from build123d import *

# Parameters (mm, degrees)
F1_DEPTH = 90.3440154
F2_R     = 2.0828
F3_DEPTH = 3.175
F5_DEPTH = 20.240498
F6_SIZE  = 20.240488
F7_R     = 1.7272
F8_DEPTH = 4.7625


# Not quite as in the source:
# - a fillet or chamfer is up to 0.001 mm smaller than in the source, because OpenCascade refuses the exact size


with BuildPart() as f1:
    # F0 (on Top) → F1 (new body)
    with BuildSketch(Plane.XY):
        with BuildLine():
            Line((32.7249998, 0), (0, 0))
            Line((0, 0), (0, 1.1500104))
            ThreePointArc((0, 1.1500104), (-10.675, 11.8250104), (-21.35, 1.1500104))
            Line((-21.35, 1.1500104), (-21.35, -3.175))
            Line((-21.35, -3.175), (-18.175, -3.175))
            Line((-18.175, -3.175), (-18.175, 1.1500104))
            ThreePointArc((-18.175, 1.1500104), (-10.675, 8.6500104), (-3.175, 1.1500104))
            Line((-3.175, 1.1500104), (-3.175, -3.175))
            Line((-3.175, -3.175), (35.8999998, -3.175))
            Line((35.8999998, -3.175), (35.8999998, 1.1500104))
            ThreePointArc((35.8999998, 1.1500104), (43.3999998, 8.6500104), (50.8999998, 1.1500104))
            Line((50.8999998, 1.1500104), (50.8999998, -3.175))
            Line((50.8999998, -3.175), (54.0749998, -3.175))
            Line((54.0749998, -3.175), (54.0749998, 1.1500104))
            ThreePointArc((54.0749998, 1.1500104), (43.3999998, 11.8250104), (32.7249998, 1.1500104))
            Line((32.7249998, 1.1500104), (32.7249998, 0))
        make_face()
    extrude(amount=F1_DEPTH)

    # F2 (on face) → F3 (cut, through all)
    with BuildSketch(Plane(origin=(0, 0, 0), x_dir=(-1, 0, 0), z_dir=(0, 1, 0))):
        with Locations((-3.96875, 3.96875)):
            Circle(F2_R)
        with Locations((-28.7562498, 3.96875)):
            Circle(F2_R)
        with Locations((-28.7562498, 86.3752654)):
            Circle(F2_R)
        with Locations((-3.96875, 86.3752654)):
            Circle(F2_R)
    extrude(amount=-F3_DEPTH, mode=Mode.SUBTRACT)

    # F4 (on face) → F5 (join)
    with BuildSketch(Plane(origin=(0, 0, 0), x_dir=(-1, 0, 0), z_dir=(0, 1, 0))):
        Polygon((-25.8874999, 55.52801188), (-25.8874999, 30.52501388), (-6.8374999, 30.52501388), (-6.8374999, 55.52801188), (-11.5999999, 55.52801188), (-11.5999999, 35.28751388), (-21.1249999, 35.28751388), (-21.1249999, 55.52801188), align=None)
    extrude(amount=F5_DEPTH)

    # F6 (size 20.240498 in the source; OpenCascade refuses exactly that, so slightly less here)
    f6_edges = [f1.edges().sort_by_distance(p)[0] for p in [
        (23.50625, 20.240498, 55.528012),
        (9.21875, 20.240498, 55.528012),
    ]]
    chamfer(f6_edges, length=F6_SIZE)

    # F7 (on face) → F8 (cut, through all)
    with BuildSketch(Plane.XY.offset(35.28751388)):
        with Locations((16.3624999, 15.477998)):
            Circle(F7_R)
    extrude(amount=-F8_DEPTH, mode=Mode.SUBTRACT)


solid = f1.part
Design review of the part built by this model. Coordinates are the model's own, in mm. A direction names the side the tool comes from. Round coordinates to 2 decimals unless told otherwise and drop trailing zeros. Write each loop counter-clockwise with the first axis right and the second up, starting at its lowest first coordinate (ties: lowest second). Pieces come first, ordered by that corner, then holes. Notation, with made-up numbers: (3, 57) -> (26, 57) arc R25 ccw to (26, 82) -> close; hole circle Ø5 at (11.5, 12). An arc over 180 degrees is marked (long way). One line per question, with ' | ' between items.
(1) Machinability: for faces 1 (the flat face through (50.9, -1, 45)), 2 (the flat face through (52, -3.175, 45)), 3 (the flat face through (23.47, 10.26, 45.27)), 4 (the cylindrical face through (3.01, -1.57, 2.12)), 5 (the flat face through (6.837, 8, 40)), which of the approach directions +Z, -Z, +X, -X, +Y, -Y give a long, thin tool a straight path to every point of the face, cutting with its end or side? Answer none if there is none.
Result sheet:
face 1: +Z, -Z, -Y | face 2: +Z, -Z, +X, -X, -Y | face 3: +Z, +Y | face 4: +Y, -Y | face 5: +Z, -Z, +Y
(2) Take a section at D-D, the plane x = -14. State the section outline as (y, z) points.
Result sheet:
outline: (7.87, 0) -> (11.29, 0) -> (11.29, 90.34) -> (7.87, 90.34) -> close
(3) Take a section at A-A, the plane y = 9.75. State the section outline as (x, z) points (1 decimal).
Result sheet:
outline: (-17, 0) -> (-4.4, 0) -> (-4.4, 90.3) -> (-17, 90.3) -> close; (6.8, 30.5) -> (25.9, 30.5) -> (25.9, 45.8) -> (21.1, 45.8) -> (21.1, 35.3) -> (11.6, 35.3) -> (11.6, 45.8) -> (6.8, 45.8) -> close; (37.1, 0) -> (49.7, 0) -> (49.7, 90.3) -> (37.1, 90.3) -> close
(4) Insertion check: P1, Ø12, axis at x = -4.5, y = 12, coming from the -Z side; P2, Ø5, axis at x = 17, y = 14.5, coming from the +Z side; P3, Ø9.5, axis at x = 20.5, y = 14.5, coming from the -Z side (3 decimals); P4, Ø16.5, axis at x = 21.5, z = 61, coming from the +Y side. Each pin has a flat end and moves straight along its axis. Give the tip position at first contact, or say it passes through.
Result sheet:
P1: z = 0 | P2: z = 35.29 | P3: z = 30.525 | P4: y = 2.78
(5) Draft analysis for pull direction Z (two halves, no side actions). For faces 6 (the cylindrical face through (26.832, -1.565, 3.171)), 7 (the flat face through (19, -1, 0)), 8 (the flat face through (16, -3.175, 45)), 9 (the cylindrical face through (27.795, -1.565, 84.527)), state which applies: released by +Z, released by -Z, zero draft, split by the parting line, or undercut.
Result sheet:
face 6: undercut | face 7: released by -Z | face 8: zero draft | face 9: undercut
(6) Take a section at C-C, the plane x = 43.4. State the section outline as (y, z) points.
Result sheet:
outline: (8.65, 0) -> (11.83, 0) -> (11.83, 90.34) -> (8.65, 90.34) -> close
(7) Take a section at B-B, the plane x = 28.5. State the section outline as (y, z) points (3 decimals).
Result sheet:
outline: (-3.175, 0) -> (0, 0) -> (0, 1.902) -> (-3.175, 1.902) -> close; (-3.175, 6.036) -> (0, 6.036) -> (0, 84.308) -> (-3.175, 84.308) -> close; (-3.175, 88.442) -> (0, 88.442) -> (0, 90.344) -> (-3.175, 90.344) -> close
(8) Wall thickness on line 1 (X direction, y = -1, z = 47.5) (3 decimals); line 2 (X direction, y = 0.25, z = 71) (3 decimals); line 3 (X direction, y = 4.5, z = 72.5): over which ranges is each line inside the solid? List them lowest first. Write a range as [from, to].
Result sheet:
line 1: [-21.35, -18.175], [-3.175, 35.9], [50.9, 54.075] | line 2: [-21.35, -18.175], [-3.175, 0], [32.725, 35.9], [50.9, 54.075] | line 3: [-20.81, -17.39], [-3.96, -0.54], [33.26, 36.69], [50.11, 53.54]
